Autodesk Inventor part; units mm, degrees
ref_plane "YZ Plane" through (0, 0, 0) normal (1, 0, 0) x (0, 1, 0)
ref_plane "XZ Plane" through (0, 0, 0) normal (0, 1, 0) x (-1, 0, 0)
ref_plane "XY Plane" through (0, 0, 0) normal (0, 0, 1) x (1, 0, 0)
ref_plane "Work Plane1" through (0, 0, 0) normal (0, 0, 1) x (1, 0, 0)
sketch "Sketch1" plane through (0, 0, 0) normal (0, 0, 1) x (1, 0, 0)
  line L0 (22.75, 48.75) -> (-33.25, 48.75) construction
  line L1 (-46.45, 48.75) -> (-46.45, 42.75)
  line L2 (-21.95, 42.75) -> (-26.45, 42.75)
  line L3 (-26.45, 42.75) -> (-26.45, 0.75)
  line L4 (-26.45, 0.75) -> (-21.95, 0.75)
  line L5 (-21.95, 0.75) -> (-21.95, 42.75)
  line L6 (-46.45, 49) -> (-46.45, 41.0784) construction
  line L7 (-46.45, 42.75) -> (-2.25, 42.75)
  line L8 (-2.25, 42.75) -> (-2.25, 48.75)
  line L9 (-2.25, 48.75) -> (-46.45, 48.75)
  line L10 (22.75, -48.75) -> (22.75, 48.75) construction
  point P0 (0, 0)
  dimension "d1" = 20
  dimension "d2" = 4.5
  dimension "d23" = 25
  dimension "d24" = 6
  dimension "d25" = 48
extrude "Extrusion1" add sketch "Sketch1" along normal blind 25
chamfer "Chamfer2" distance 25 angle 3.5 1 edges at (-26.45, 21.75, 25) measured on face at (-26.45, 28.75, 8.3333)
sketch "Sketch2" plane through (-26.45, 0.75, 0) normal (-0.9981348, 0, 0.0610485) x (0.0610485, 0, 0.9981348)
  line L0 (0, 0) -> (25.0467, 0) construction
  line L1 (0, 42) -> (0, 0) construction
  line L2 (9.75, 39) -> (9.75, 3) construction
  point P0 (1.6147, -0.75)
  point P1 (9.75, 21)
  point P2 (0, 21)
  dimension "d12" = 36
  dimension "d13" = 9.75
hole "Hole1" at (-25.8548, 39.75, 9.7318) at (-25.8548, 3.75, 9.7318) direction (0.9981348, 0, -0.0610485) diameter 4 depth 4 counterbore diameter 4.5 counterbore depth 0.6
sketch "Sketch4" plane through (-2.25, 48.75, 25) normal (0, 1, 0) x (1, 0, 0)
  circle A0 centre (10.5, 12.5) radius 12.2 construction
  circle A1 centre (10.5, 12.5) radius 12.4
  dimension "d42" = 0.2
extrude "Extrusion3" cut sketch "Sketch4" against normal through all
sketch "Sketch5" plane through (0, 0, 25) normal (0, 0, 1) x (1, 0, 0)
  line L0 (-46.45, 48.75) -> (-46.45, 42.75)
  line L1 (-2.25, 48.75) -> (-46.45, 48.75)
  line L2 (-46.45, 48.75) -> (-46.45, 47.25)
  line L3 (-46.45, 47.25) -> (-2.25, 47.25)
  line L4 (-2.25, 47.25) -> (-2.25, 48.75)
  point P0 (0, 0)
  dimension "d29" = 1.5
extrude "Extrusion4" add sketch "Sketch5" along normal blind 2
sketch "Sketch3" plane through (22.75, 48.75, 25) normal (0, 1, 0) x (1, 0, 0)
  line L0 (-69.2, 23) -> (-64.5, 23)
  line L1 (-64.5, 23) -> (-64.5, 25)
  line L2 (-64.5, 25) -> (-69, 25)
  line L3 (-69, 25) -> (-69, 27.5)
  line L4 (-69, 27.5) -> (-73.7, 27.5)
  line L5 (-73.7, 27.5) -> (-69.2, 23)
  line L6 (-64.3, 22.8) -> (-69.2828, 22.8)
  line L7 (-69.2828, 22.8) -> (-74.1828, 27.7)
  line L8 (-74.1828, 27.7) -> (-68.8, 27.7)
  line L9 (-68.8, 27.7) -> (-68.8, 25.2)
  line L10 (-68.8, 25.2) -> (-64.3, 25.2)
  line L11 (-64.3, 25.2) -> (-64.3, 22.8)
  line L12 (-69.2, 25) -> (-69.2, -2)
  line L13 (-69.2, 22.8) -> (-54.8817, -2)
  line L14 (-54.8817, -2) -> (-69.2, -2)
  line L15 (-69.2, -2) -> (-69.2, 22.8)
  line L16 (-54.8817, -2) -> (-53.4961, -2)
  line L17 (-25, -2) -> (-69.2, -2)
  line L18 (-67.8144, 22.8) -> (-53.4961, -2)
  point P0 (-22.75, 25)
  point P1 (-68.85, 25.15)
  point P2 (-68.7, 25)
  dimension "d32" = 0.2
  dimension "d33" = 30
  dimension "d34" = 1.2
extrude "Extrusion2" cut sketch "Sketch3" against normal through all contours L5 L4 L3 L2 L1 L0 | L6 L7 L8 L9 L10 L11 | L18 L16 L13 L6 | L13 L14 L12
sketch "Sketch6" plane through (0, 0, 0) normal (0, 0, -1) x (-1, 0, 0)
  arc A0 (7.2895, 48.75) -> (9.2105, 48.75) centre (8.25, 45.75) ccw construction
  arc A1 (29.2895, 48.75) -> (33.25, 44.7895) centre (30.25, 45.75) ccw construction
  point P0 (0, 0)
hole "Hole2" at (-8.25, 45.75, 0) at (-30.25, 45.75, 0) direction (0, 0, 1) diameter 4 depth 4 counterbore diameter 4.5 counterbore depth 0.6
sketch "Sketch7" plane through (0, 0, 25) normal (0, 0, 1) x (1, 0, 0)
  line L0 (-2.25, 42.75) -> (-2.25, 47.25) construction
  line L1 (-31.9008, 47.25) -> (-31.9008, 42.75) construction
  point P0 (0, 0)
  point P1 (-6.25, 45)
  point P2 (-27.9008, 45)
  point P3 (-2.25, 45)
  point P4 (-2.25, 45)
  dimension "d43" = 4
  dimension "d44" = 4
hole "Hole3" at (-27.9008, 45, 25) at (-6.25, 45, 25) direction (0, 0, -1) diameter 4 depth 4 counterbore diameter 4.5 counterbore depth 0.6
sketch "Sketch8" plane through (-2.25, 42.75, 19.0962) normal (1, 0, 0) x (0, 0, -1)
  line L0 (-5.9038, 0) -> (19.0962, 0)
  line L1 (-1.4038, 0) -> (-5.9038, -2)
  line L2 (-5.9038, -42) -> (-5.9038, 0)
  line L3 (-5.9038, 0) -> (-5.9038, -2)
  point P0 (19.0962, -42.75)
  dimension "d52" = 4.5
  dimension "d53" = 2
extrude "Extrusion5" add sketch "Sketch8" against normal up to surface surface through (-45.0644, 48.75, 2.2) normal (0.8660254, 0, -0.5)
properties part number "bok"
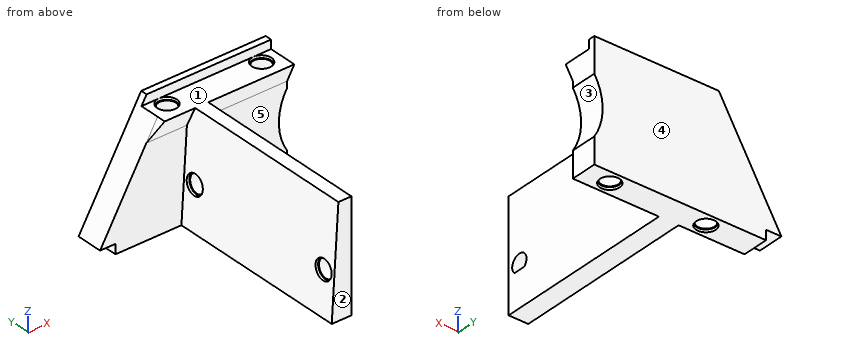
Verification items for the finished model (mm, model axes). Face numbers are marked on the shaded views. A direction names the side the tool comes from. Coordinates: 2 decimals unless noted, no trailing zeros. Write each loop counter-clockwise with the first axis right and the second up, starting at its lowest first coordinate (ties: lowest second). Pieces come first, ordered by that corner, then holes. Notation, with made-up numbers: M -9.5,56.5 L -2.5,56.5 A8 ccw -2.5,66.5 Z; hole C 73,50 d11. An arc over 180 degrees is marked long. Answer as a JSON object with one key per item and string values. Group by question number.
(1) Gauge pin test, flat ends, axial feed: pin 1 (2 mm diameter, centred on x = -28, y = 45, fed in from +Z); pin 2 (1 mm diameter, centred on x = -10, z = 19, fed in from -Y); pin 3 (5 mm diameter, centred on y = 37.5, z = 14, fed in from +X). Record the tip position at first contact, or that the pin passes through.
(2) Cross-section at B-B, the plane x = -20. Record the cut outline in (y, z), and give its area (4 significant figures).
(3) Tool access check on the marked faces 4 and 5. Record the directions out of +Z, -Z, +X, -X, +Y, -Y that give a thin tool (end or side, any length) a straight path to the whole face; none if there is none.
(4) Release check for a two-part mould opening along Z. For the marked faces 1, 2 and 3 record: +Z half, -Z half, draft (parallel to the pull), parting line (faces both ways), or undercut.
(5) Material ranges on line 1 (X direction, y = 45.75, z = 0.3); line 2 (X direction, y = 45.75, z = 2.45); line 3 (Y direction, x = -30.25, z = 1.5), recorded low to high.
(6) Cross-section at D-D, the plane x = -40.5. Record the cut outline in (y, z), and give its area (3 significant figures).
(7) Cross-section at C-C, the plane z = 14.5. Record the cut outline in (x, y), and give its area (3 significant figures).
Reply:
{
 "1": {"pin 1": "z = 21", "pin 2": "y = 42.75", "pin 3": "x = -21.95"},
 "2": {"outline": "M 40.75,25 L 42.75,20.5 L 42.75,0 L 48.75,0 L 48.75,27 L 47.25,27 L 47.25,25 Z", "area": "157.5 mm²"},
 "3": {"face 4": "+Z, -Z, +X, -X, +Y", "face 5": "-Z, +X, -Y"},
 "4": {"face 1": "+Z half", "face 2": "draft", "face 3": "undercut"},
 "5": {"line 1": "-41.55 to -32.5, -28 to -10.5, -6 to -2.25", "line 2": "-44.92 to -32.25, -28.25 to -10.25, -6.25 to -2.25", "line 3": "42.75 to 43.75, 47.75 to 48.75"},
 "6": {"outline": "M 42.75,0 L 48.75,0 L 48.75,10.11 L 42.75,10.11 Z", "area": "60.6 mm²"},
 "7": {"outline": "M -37.96,42.75 L -25.56,42.75 L -25.56,0.75 L -21.95,0.75 L -21.95,42.75 L -3.99,42.75 L -3.99,48.75 L -37.96,48.75 Z", "area": "356 mm²"}
}
